Autodesk Inventor part; units mm, degrees
ref_plane "YZ Plane" through (0, 0, 0) normal (1, 0, 0) x (0, 1, 0)
ref_plane "XZ Plane" through (0, 0, 0) normal (0, 1, 0) x (-1, 0, 0)
ref_plane "XY Plane" through (0, 0, 0) normal (0, 0, 1) x (1, 0, 0)
sketch "Sketch1" plane through (0, 0, 0) normal (0, 1, 0) x (-1, 0, 0)
  line L0 (8.4436, 19.7296) -> (-51.5564, 19.7296)
  line L1 (-51.5564, 19.7296) -> (-51.5564, -26.2704)
  line L2 (-51.5564, -26.2704) -> (8.4436, -26.2704)
  line L3 (8.4436, -26.2704) -> (8.4436, 19.7296)
  point P0 (0, 0)
  dimension "d0" = 60
  dimension "d1" = 46
extrude "Extrusion1" add sketch "Sketch1" along normal blind 3.7
sketch "Sketch2" plane through (0, 3.7, 0) normal (0, 1, 0) x (1, 0, 0)
  line L0 (-8.4436, -19.7296) -> (51.5564, -19.7296)
  line L1 (-8.4436, 26.2704) -> (-8.4436, -19.7296)
  line L2 (51.5564, -19.7296) -> (51.5564, 26.2704)
  line L3 (-8.4436, -19.7296) -> (-0.0236, -19.7296)
  line L4 (51.5564, -19.7296) -> (45.1564, -19.7296)
  line L5 (45.1564, -19.7296) -> (45.1564, -14.2296)
  line L6 (45.1564, -14.2296) -> (-0.0236, -14.2296)
  line L7 (-0.0236, -14.2296) -> (-0.0236, -24.2296)
  line L8 (-0.0236, -24.2296) -> (45.1564, -24.2296)
  line L9 (45.1564, -24.2296) -> (45.1564, -14.2296)
  point P0 (0, 0)
  dimension "d4" = 8.42
  dimension "d5" = 6.4
  dimension "d6" = 5.5
  dimension "d7" = 10
extrude "Extrusion2" add sketch "Sketch2" along normal blind 17.6
sketch "Sketch3" plane through (0, 3.7, 0) normal (0, 1, 0) x (1, 0, 0)
  line L0 (-8.4436, 26.2704) -> (-8.4436, -19.7296)
  line L1 (-2.3236, 26.2704) -> (-2.3236, -19.7296)
  line L2 (45.1564, -14.2296) -> (-0.0236, -14.2296)
  line L3 (45.1564, -12.5296) -> (-0.0236, -12.5296)
  line L4 (-2.3236, -12.5296) -> (23.6764, -12.5296)
  line L5 (23.6764, -12.5296) -> (23.6764, 13.9704)
  line L6 (23.6764, 13.9704) -> (-2.3236, 13.9704)
  line L7 (-2.3236, 13.9704) -> (-2.3236, -12.5296)
  point P0 (0, 0)
  dimension "d10" = 6.12
  dimension "d11" = 1.7
  dimension "d12" = 26
  dimension "d13" = 26.5
extrude "Extrusion3" add sketch "Sketch3" along normal blind 13.9
sketch "Sketch4" plane through (0, 3.7, 0) normal (0, 1, 0) x (1, 0, 0)
  line L0 (-8.4436, -19.7296) -> (-0.0236, -19.7296)
  line L1 (-6.5036, 26.2704) -> (-6.5036, -17.7896)
  line L2 (-0.0236, -18.3496) -> (-7.0636, -18.3496)
  circle A0 centre (-5.0036, -16.8496) radius 1.5
  line L3 (51.5564, 26.2704) -> (-8.4436, 26.2704)
  line L4 (51.5564, 24.8704) -> (-7.0436, 24.8704)
  circle A1 centre (-5.0036, 23.3704) radius 1.5
  line L5 (49.7164, -19.7296) -> (49.7164, 24.4304)
  line L6 (-0.0236, -41.0522) -> (-29.7662, -41.0522)
  line L7 (-29.7662, -41.0522) -> (-29.7662, 47.593)
  line L8 (-29.7662, 47.593) -> (72.879, 47.593)
  line L9 (72.879, 47.593) -> (72.879, -19.7296)
  line L10 (45.1564, -19.7296) -> (51.5564, -19.7296)
  line L11 (45.1564, -18.2796) -> (50.1064, -18.2796)
  circle A2 centre (48.2164, -16.7796) radius 1.5
  line L12 (51.5564, 14.4704) -> (-7.0436, 14.4704)
  circle A3 centre (48.2164, 12.9704) radius 1.5
  point P0 (0, 0)
  dimension "d17" = 1.38
  dimension "d18" = 3
  dimension "d19" = 1.4
  dimension "d20" = 3
  dimension "d22" = 1.45
  dimension "d23" = 3
  dimension "d24" = 10.4
  dimension "d25" = 3
extrude "Extrusion4" cut sketch "Sketch4" against normal blind 13.9 contours A2 | A3 | A0 | A1
sketch "Sketch5" plane through (0, 0, 0) normal (0, -1, 0) x (1, 0, 0)
  line L0 (51.5564, 19.7296) -> (51.5564, -26.2704)
  line L1 (-8.4436, 19.7296) -> (51.5564, 19.7296)
  line L2 (-8.4436, -26.2704) -> (-8.4436, 19.7296)
  line L3 (51.5564, -26.2704) -> (-8.4436, -26.2704)
  line L4 (43.9969, -18.7109) -> (43.9969, 12.1701)
  line L5 (43.9969, 12.1701) -> (-0.8841, 12.1701)
  line L6 (-0.8841, 12.1701) -> (-0.8841, -18.7109)
  line L7 (-0.8841, -18.7109) -> (43.9969, -18.7109)
  point P0 (0, 0)
extrude "Extrusion5" cut sketch "Sketch5" against normal blind 2.65
sketch "Sketch6" plane through (0, 3.7, 0) normal (0, 1, 0) x (1, 0, 0)
  line L0 (51.5564, -19.7296) -> (51.5564, 26.2704)
  line L1 (48.3964, -19.7296) -> (48.3964, 26.2704)
  line L2 (51.5564, 26.2704) -> (-8.4436, 26.2704)
  line L3 (48.3964, 26.2704) -> (13.2964, 26.2704)
  line L4 (13.2964, 26.2704) -> (13.2964, 16.2704)
  line L5 (13.2964, 16.2704) -> (48.3964, 16.2704)
  line L6 (48.3964, 16.2704) -> (48.3964, 26.2704)
  point P0 (0, 0)
  dimension "d30" = 3.16
  dimension "d31" = 35.1
  dimension "d32" = 10
extrude "Extrusion6" add sketch "Sketch6" along normal blind 12.5
properties part number "CapCharger"
Input: part model. Units: mm. Frame: model coordinates. A direction names the side the tool comes from. Give positions to 0.01 mm unless a question says otherwise; leave off trailing zeros. Order: outer loops, then holes, each group sorted by start corner. A loop starts at its lowest first (then second) coordinate and runs counter-clockwise, first axis right, second up. Notation, with made-up numbers: (12, 56) - (32, 56) arc R21 cw to (32, 69) - close; hole circle Ø1 at (82, 63.5). An arc over 180 degrees is marked (long way). Answer as a JSON object with one key per item and string values. Group by question number.
Q1. Line query: probe 1 along Z at (x, y) = (33, 14); probe 2 along Z at (x, y) = (5, 11); probe 3 along X at (y, z) = (6.25, -8.5). Output: solid intervals per line, ascending.
Q2. Mould query, pull axis X, two halves, no side actions, for faces 1 (the face through (31, 16.2, -21)), 2 (the face through (48.396, 10, -21)), 3 (the face through (49.647, 3.182, 16.329)), 4 (the face through (-5.329, 3.182, 18.314)). Classes: pulls with the +X half, pulls with the -X half, needs draft (parallel to the pull), parting line crosses it, or undercut.
Q3. First-contact query: pin 1 Ø13 at (x, z) = (12.5, 2.5) entering from +Y; pin 2 Ø4 at (x, y) = (2.5, 15.5) entering from -Z; pin 3 Ø3 at (y, z) = (1, 0.5) entering from +X; pin 4 Ø1.8 at (x, z) = (-5, -23.37) entering from -Y. Flat tips, straight axial feed; report the tip coordinate or a pass-through.
Q4. Cut plane A-A, the plane y = 11.25. Output: boundary loops of the cut face in (x, z), then the cut area to 3 significant figures.
Q5. Cut plane D-D, the plane x = 14. Output: boundary loops of the cut face in (y, z).
Q6. Cut plane B-B, the plane x = 28.5. Output: boundary loops of the cut face in (y, z), then the cut area to 3 significant figures.
Q7. Set-up query: faces 5 (the face through (22, 1, 12.17)), 6 (the face through (-0.884, 1, -3)), 7 (the face through (10, 11, 12.53)), 8 (the face through (-2.324, 11, -1)). Return all of +Z, -Z, +X, -X, +Y, -Y with unobstructed straight access to the full face (end or side cutting, diameter ignored); none if empty.
Q8. Cut plane C-C, the plane z = 11.5. Output: boundary loops of the cut face in (x, y).
Results:
{
 "1": {"probe 1": "-26.27 to -16.27, 14.23 to 24.23", "probe 2": "-13.97 to 12.53, 14.23 to 24.23", "probe 3": "-2.32 to 23.68"},
 "2": {"face 1": "needs draft", "face 2": "pulls with the +X half", "face 3": "undercut", "face 4": "undercut"},
 "3": {"pin 1": "y = 17.6", "pin 2": "z = -13.97", "pin 3": "x = 44", "pin 4": "through"},
 "4": {"outline": "(-2.32, -13.97) - (23.68, -13.97) - (23.68, 12.53) - (-2.32, 12.53) - close; (-0.02, 14.23) - (45.16, 14.23) - (45.16, 24.23) - (-0.02, 24.23) - close; (13.3, -26.27) - (48.4, -26.27) - (48.4, -16.27) - (13.3, -16.27) - close", "area": "1,490 mm^2"},
 "5": {"outline": "(0, -18.71) - (2.65, -18.71) - (2.65, -26.27) - (16.2, -26.27) - (16.2, -16.27) - (3.7, -16.27) - (3.7, -13.97) - (17.6, -13.97) - (17.6, 12.53) - (3.7, 12.53) - (3.7, 14.23) - (21.3, 14.23) - (21.3, 24.23) - (3.7, 24.23) - (3.7, 19.73) - (2.65, 19.73) - (2.65, 12.17) - (0, 12.17) - close"},
 "6": {"outline": "(0, -18.71) - (2.65, -18.71) - (2.65, -26.27) - (16.2, -26.27) - (16.2, -16.27) - (3.7, -16.27) - (3.7, 14.23) - (21.3, 14.23) - (21.3, 24.23) - (3.7, 24.23) - (3.7, 19.73) - (2.65, 19.73) - (2.65, 12.17) - (0, 12.17) - close", "area": "431 mm^2"},
 "7": {"face 5": "+Z, +X, -X, -Y", "face 6": "+Z, -Z, -X, -Y", "face 7": "+X, -X, +Y", "face 8": "+Z, -Z, -X, +Y"},
 "8": {"outline": "(-8.44, 2.65) - (-0.88, 2.65) - (-0.88, 0) - (44, 0) - (44, 2.65) - (51.56, 2.65) - (51.56, 3.7) - (23.68, 3.7) - (23.68, 17.6) - (-2.32, 17.6) - (-2.32, 3.7) - (-8.44, 3.7) - close"}
}
